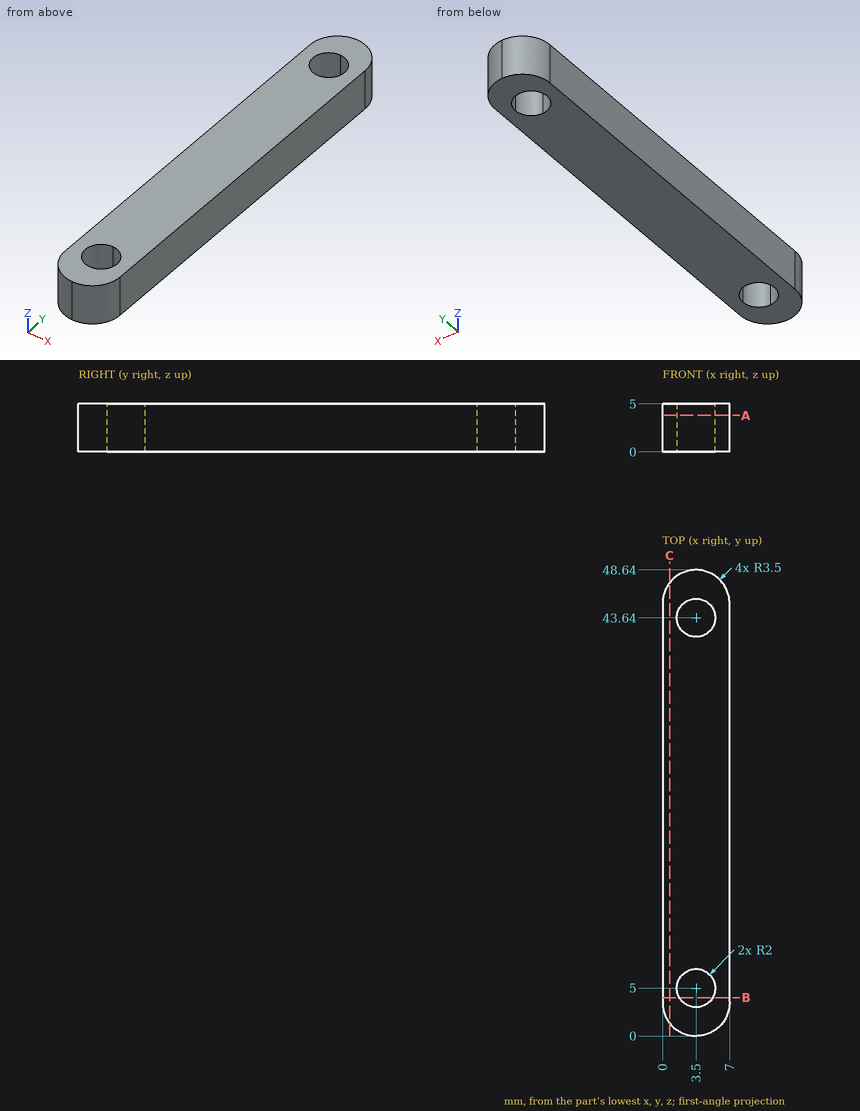
Study the drawing (mm; zero at the part's minimum x, y, z) and answer. Give positions to 0.01 mm unless a question says otherwise; leave off trailing zeros. Order: outer loops, then holes, each group sorted by start corner. A loop starts at its lowest first (then second) coordinate and runs counter-clockwise, first axis right, second up.
1. This flat-tipped pin is pushed along its axis until it touches: P1, Ø3, axis at x = 6, z = 3.5, coming from the -Y side. Where does it stop, or does it pass through?
Result sheet:
P1: stops at y = 0.15
2. Straight lines are drawn through the part: L1, parallel to Y at x = 2, z = 1.6; L2, parallel to Y at x = 3.75, z = 4.55; L3, parallel to X at y = 45, z = 2.8. For each, find the intervals that lie inside material, in ascending order.
Result sheet:
L1: y = 0.34 to 3.68, 6.32 to 42.32, 44.96 to 48.3
L2: y = 0.01 to 3.02, 6.98 to 41.66, 45.62 to 48.63
L3: x = 0 to 2.03, 4.97 to 7
3. Section C-C, the plane x = 0.75 is taken. Determine the outline of the cut face in (y, z) (3 decimals).
Result sheet:
outline: (1.335, 0) - (47.305, 0) - (47.305, 5) - (1.335, 5) - close
4. Section A-A, the plane z = 3.8 is taken. Give the number of separate pieces and of enclosed holes in the cut face, and give its area (3 significant figures).
Result sheet:
separate pieces: 1
enclosed holes: 2
area: 305 mm2
5. Section B-B, the plane y = 4 is taken. Determine the outline of the cut face in (x, z), and give its area (3 significant figures).
Result sheet:
outline: (0, 0) - (1.77, 0) - (1.77, 5) - (0, 5) - close; (5.23, 0) - (7, 0) - (7, 5) - (5.23, 5) - close
area: 17.7 mm2
